Verification items for the finished model (mm, model axes). Coordinates: 2 decimals unless noted, no trailing zeros. Write each loop counter-clockwise with the first axis right and the second up, starting at its lowest first coordinate (ties: lowest second). Pieces come first, ordered by that corner, then holes. Notation, with made-up numbers: (73.25, 61) - (81.25, 61) arc R16 cw to (81.25, 78) - close; hole circle Ø8 at (66, 66). An arc over 180 degrees is marked (long way). Use one line per item in the form item = value. Start each with the question number.
(1) Sectioned sample at B-B (x = -11). Record the cut outline in (y, z).
(2) Sectioned sample at A-A (z = 6.5). Record the cut outline in (x, y).
(3) Gauge pin test, flat ends, axial feed: pin 1 Ø1.5 at (x, z) = (-14, 43) entering from -Y; pin 2 Ø10 at (x, z) = (0.5, 32.5) entering from +Y; pin 3 Ø3 at (x, z) = (6.5, 48.5) entering from -Y. Record the tip position at first contact, or that the pin passes through.
(4) Material ranges on line 1 (Y direction, x = -2.5, z = 30); line 2 (Y direction, x = -7, z = 34.5); line 3 (Z direction, x = -4, y = 97), recorded low to high. Write a range as [from, to].
from build123d import *

# Parameters (mm, degrees)
F0_W     = 35
F0_H     = 240
F1_DEPTH = 3
F2_W     = 240
F2_H     = 55
F3_DEPTH = 22.5
F5_DEPTH = 45.001


with BuildPart() as f1:
    # F0 (on Top) → F1 (new body)
    with BuildSketch(Plane.XY):
        Rectangle(F0_W, F0_H)
    extrude(amount=F1_DEPTH)

    # F2 (on Right) → F3 (join, symmetric)
    with BuildSketch(Plane.YZ):
        with Locations((0, 27.5)):
            Rectangle(F2_W, F2_H)
    extrude(amount=F3_DEPTH, both=True)

    # F4 (on face) → F5 (cut, through all)
    with BuildSketch(Plane.YZ.offset(22.5)):
        Polygon((-120, 55), (-120, 0), (-78.704832, 55), align=None)
        Polygon((78.704832, 55), (120, 0), (120, 55), align=None)
    extrude(amount=-F5_DEPTH, mode=Mode.SUBTRACT)


solid = f1.part
Answers below:
q1.outline = (-120, 0) - (120, 0) - (78.7, 55) - (-78.7, 55) - close
q2.outline = (-22.5, -115.12) - (22.5, -115.12) - (22.5, 115.12) - (-22.5, 115.12) - close
q3.pin_1 = -88.28
q3.pin_2 = 99.35
q3.pin_3 = -84.71
q4.line_1 = [-97.48, 97.48]
q4.line_2 = [-94.1, 94.1]
q4.line_3 = [0, 30.63]
